Design review of the part shown in the three views and the two pictorial views. Dimensions are in mm from the part's minimum x, y and z. Give positions to 0.01 mm unless a question says otherwise; leave off trailing zeros. Loops run counter-clockwise (first coordinate to the right, second up) from the corner with the lowest first, then second, coordinate; pieces in that order, holes last. Notation, with made-up numbers: (-18, 89) -> (-5, 89) arc R26 cw to (-5, 124) -> close; hole circle Ø7 at (-24.5, -15). An arc over 180 degrees is marked (long way). One line per question, with ' | ' between items. Start each with the question number.
(1) Wall thickness on probe 1 along X at (y, z) = (0.95, 1.4); probe 2 along X at (y, z) = (2.9, 3.4); probe 3 along Z at (x, y) = (10, 0.2): over which ranges is each line inside the solid? List them lowest first.
(2) Insertion check: P1, Ø1, axis at x = 4.5, z = 1, coming from the -Y side; P2, Ø1.5, axis at y = 1, z = 3.5, coming from the +X side. Each pin has a flat end and moves straight along its axis. Give the tip position at first contact, or say it passes through.
(3) Consider section A-A (z = 3.15). Write out the cut boundary in (x, y), and give its area (3 significant figures).
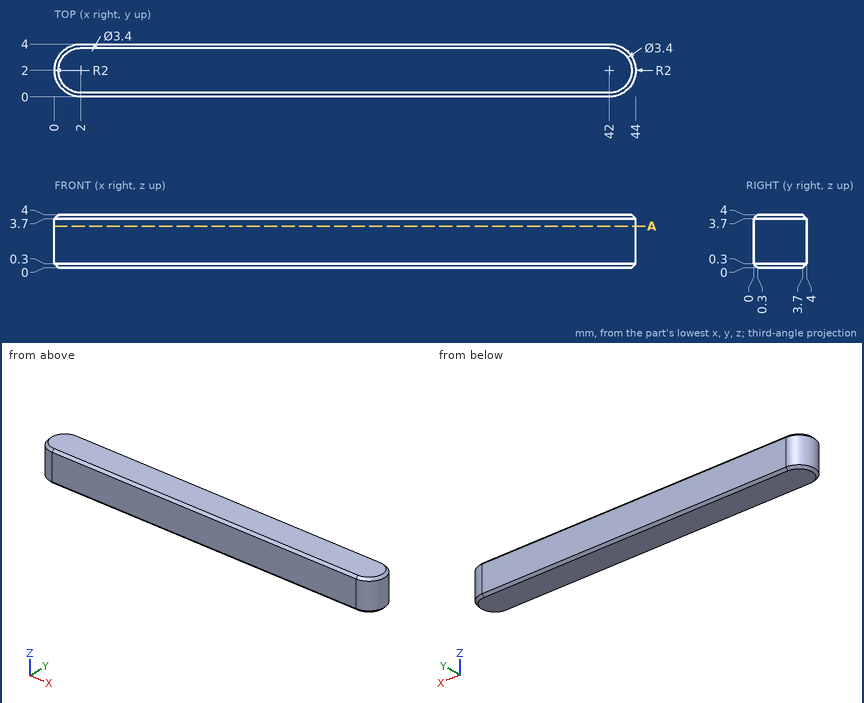
A:
1) probe 1: x = 0.3 to 43.7 | probe 2: x = 0.21 to 43.79 | probe 3: z = 0.1 to 3.9
2) P1: stops at y = 0 | P2: stops at x = 43.98
3) outline: (2, 0) -> (42, 0) arc R2 ccw to (42, 4) -> (2, 4) arc R2 ccw to start | area: 173 mm^2
